Design review of the part built by this model. Coordinates are the model's own, in mm. A direction names the side the tool comes from. Give positions to 0.01 mm unless a question says otherwise; leave off trailing zeros. Order: outer loops, then holes, each group sorted by start corner. A loop starts at its lowest first (then second) coordinate and runs counter-clockwise, first axis right, second up. Notation, with made-up numbers: (-36, -2.5) -> (-12, -2.5) arc R20 ccw to (-12, 36.5) -> close; hole circle Ø4 at (-14.75, -28). An arc over 180 degrees is marked (long way). Return JSON: item names as keys, results as strings.
```python
from build123d import *

# Parameters (mm, degrees)
SKETCH1_W                                      = 9
SKETCH1_H                                      = 12
EXTRUDE1_DEPTH                                 = 2.175
SKETCH3_W                                      = 6.9
SKETCH3_H                                      = 6.9
EXTRUDE3_DEPTH                                 = 1
CBORE_FOR_0_SOCKET_HEAD_CAP_SCREW1_D           = 1.778
CBORE_FOR_0_SOCKET_HEAD_CAP_SCREW1_CBORE_D     = 3.175
CBORE_FOR_0_SOCKET_HEAD_CAP_SCREW1_CBORE_DEPTH = 1.524
F_3_32_0_09375_DIAMETER_HOLE1_D                = 2.38125
F_3_32_0_09375_DIAMETER_HOLE1_DEPTH            = 10
F_3_32_0_09375_DIAMETER_HOLE1_TIP              = 0.715399675
FILLET1_R                                      = 1


with BuildPart() as part:
    # Sketch1 → Extrude1 (new body)
    with BuildSketch(Plane(origin=(0, 0, 0), x_dir=(1, 0, 0), z_dir=(0, 1, 0))):
        Rectangle(SKETCH1_W, SKETCH1_H)
    extrude(amount=EXTRUDE1_DEPTH)

    # Sketch3 → Extrude3 (add)
    with BuildSketch(Plane(origin=(0, 2.175, 0), x_dir=(1, 0, 0), z_dir=(0, 1, 0))):
        with Locations((0, -1.5)):
            Rectangle(SKETCH3_W, SKETCH3_H)
    extrude(amount=EXTRUDE3_DEPTH)

    # CBORE for #0 Socket Head Cap Screw1 (through all)
    with Locations(Plane(origin=(0, 0, -4), x_dir=(0, 0, -1), z_dir=(0, -1, 0))):
        with Locations((0, 0)):
            CounterBoreHole(CBORE_FOR_0_SOCKET_HEAD_CAP_SCREW1_D / 2, CBORE_FOR_0_SOCKET_HEAD_CAP_SCREW1_CBORE_D / 2, CBORE_FOR_0_SOCKET_HEAD_CAP_SCREW1_CBORE_DEPTH)

    # 3/32 (0.09375) Diameter Hole1
    with Locations(Plane(origin=(-2.5, 0, -4), x_dir=(0, 0, -1), z_dir=(0, -1, 0))):
        with Locations((0, 0), (0, 5)):
            Hole(F_3_32_0_09375_DIAMETER_HOLE1_D / 2, depth=F_3_32_0_09375_DIAMETER_HOLE1_DEPTH)
            with Locations((0, 0, -(F_3_32_0_09375_DIAMETER_HOLE1_DEPTH + F_3_32_0_09375_DIAMETER_HOLE1_TIP / 2))):  # 118° drill point
                Cone(0, F_3_32_0_09375_DIAMETER_HOLE1_D / 2, F_3_32_0_09375_DIAMETER_HOLE1_TIP, mode=Mode.SUBTRACT)

    # Fillet1
    fillet1_edges = [part.edges().sort_by_distance(p)[0] for p in [
        (-3.45, 2.675, -1.95),
        (-3.45, 2.675, 4.95),
        (3.45, 2.675, 4.95),
        (3.45, 2.675, -1.95),
        (-4.5, 1.0875, -6),
        (4.5, 1.0875, -6),
        (4.5, 1.0875, 6),
        (-4.5, 1.0875, 6),
    ]]
    fillet(fillet1_edges, radius=FILLET1_R)


solid = part.part
```
Item 1: For pin 1 (1.1 mm diameter, centred on x = 0, z = -4, fed in from -Y); pin 2 (0.8 mm diameter, centred on x = -1, y = 3, fed in from -Z); pin 3 (0.9 mm diameter, centred on x = 0, z = -5, fed in from -Y), all flat-tipped, find the tip position at first contact; note any pin that passes through.
Result set:
{"pin 1": "passes through", "pin 2": "stops at z = -1.95", "pin 3": "stops at y = 1.52"}
Item 2: Add section D-D (x = 3). Give the boundary of the cut face in (y, z) (3 decimals).
Result set:
{"outline": "(0, -6) -> (2.175, -6) -> (2.175, -5.081) -> (0, -5.081) -> close; (0, -2.919) -> (2.175, -2.919) -> (2.175, -1.785) -> (3.175, -1.785) -> (3.175, 4.785) -> (2.175, 4.785) -> (2.175, 6) -> (0, 6) -> close"}
Item 3: Machinability: for faces 4 (the face through (0.026, 0.751, -2.413)), 5 (the face through (0, 3, -1.95)), 6 (the face through (-3.45, 3, 2)), 7 (the face through (-3.165, 2.682, 4.649)), which of the approach directions +Z, -Z, +X, -X, +Y, -Y give a long, thin tool a straight path to every point of the face, cutting with its end or side? Answer none if there is none.
Result set:
{"face 4": "-Y", "face 5": "-Z, +X, -X, +Y", "face 6": "+Z, -Z, -X, +Y", "face 7": "+Z, -X, +Y"}
Item 4: Add section C-C (z = 1.75). Give the boundary of the cut face in (x, y) (3 decimals).
Result set:
{"outline": "(-4.5, 0) -> (4.5, 0) -> (4.5, 2.175) -> (3.45, 2.175) -> (3.45, 3.175) -> (-3.45, 3.175) -> (-3.45, 2.175) -> (-4.5, 2.175) -> close"}
Item 5: Mouldability with a two-part tool opening along X and no side actions: class faces 1 (the face through (-3.66, 1.1, -4.26)), 2 (the face through (-3.149, 2.682, -1.665)), 3 (the face through (0, 3.175, 1)) as released by +X, released by -X, zero draft, split by the parting line, or undercut.
Result set:
{"face 1": "undercut", "face 2": "released by -X", "face 3": "zero draft"}
Item 6: Add section A-A (z = -4). Give the boundary of the cut face in (x, y) (3 decimals), plus the area to 3 significant figures.
Result set:
{"outline": "(-4.5, 0) -> (-3.691, 0) -> (-3.691, 2.175) -> (-4.5, 2.175) -> close; (-1.309, 1.524) -> (-0.889, 1.524) -> (-0.889, 2.175) -> (-1.309, 2.175) -> close; (0.889, 1.524) -> (1.309, 1.524) -> (1.309, 2.175) -> (0.889, 2.175) -> close; (3.691, 0) -> (4.5, 0) -> (4.5, 2.175) -> (3.691, 2.175) -> close", "area": "4.07 mm^2"}
Item 7: Wall thickness on L1, parallel to Z at x = -2.5, y = 0.75; L2, parallel to X at y = 1.75, z = -4; L3, parallel to X at y = 1.1, z = -4: over which ranges is each line inside the solid? List them lowest first. Write a range as [from, to].
Result set:
{"L1": "z = [-6, -5.19], [-2.81, 6]", "L2": "x = [-4.5, -3.69], [-1.31, -0.89], [0.89, 1.31], [3.69, 4.5]", "L3": "x = [-4.5, -3.69], [3.69, 4.5]"}
